from build123d import *

# Parameters (mm, degrees)
CROQUIS3_R              = 0.5
CORTAR_EXTRUIR1_DEPTH   = 1
SALIENTE_EXTRUIR3_START = 5
SALIENTE_EXTRUIR3_DEPTH = 5


with BuildPart() as part:
    # Croquis2 → Revolución1 (revolve)
    with BuildSketch(Plane(origin=(0, 0, 0), x_dir=(0, 0, -1), z_dir=(1, 0, 0)), mode=Mode.PRIVATE) as revoluci_n1_sk:
        Polygon((0, 0), (0, 6.5), (-0.95, 6.5), (-0.95, 6.4), (-1.05, 6.4), (-1.05, 6.5), (-4, 6.5), (-4, 3.5), (-5, 3.5), (-5, 2), (-8, 2), (-8, 1.75), (-4, 1.75), (-4, 0), align=None)
    revolve(revoluci_n1_sk.sketch.rotate(Axis((0, 0, 4), (0, 0, -1)), 90), axis=Axis((0, 0, 4), (0, 0, -1)))

    # Croquis3 → Cortar-Extruir1 (cut)
    with BuildSketch(Plane(origin=(0, 0, 0), x_dir=(-1, 0, 0), z_dir=(0, 0, -1))):
        with Locations((-2, -3)):
            Circle(CROQUIS3_R)
        with Locations((2, -3)):
            Circle(CROQUIS3_R)
        with Locations((0, -2)):
            Circle(CROQUIS3_R)
    extrude(amount=-CORTAR_EXTRUIR1_DEPTH, mode=Mode.SUBTRACT)

    # Croquis5 → Saliente-Extruir3 (add)
    with BuildSketch(Plane(origin=(0, 0, 1), x_dir=(-1, 0, 0), z_dir=(0, 0, -1)).offset(SALIENTE_EXTRUIR3_START)):
        with BuildLine():
            Line((-0.489897949, -1.9), (0.489897949, -1.9))
            ThreePointArc((0.489897949, -1.9), (0.5, -2), (0.489897949, -2.1))
            Line((0.489897949, -2.1), (-0.489897949, -2.1))
            ThreePointArc((-0.489897949, -2.1), (-0.5, -2), (-0.489897949, -1.9))
        make_face()
        with BuildLine():
            Line((1.510102051, -2.9), (2.489897949, -2.9))
            ThreePointArc((2.489897949, -2.9), (2.5, -3), (2.489897949, -3.1))
            Line((2.489897949, -3.1), (1.510102051, -3.1))
            ThreePointArc((1.510102051, -3.1), (1.5, -3), (1.510102051, -2.9))
        make_face()
        with BuildLine():
            Line((-2.489897949, -2.9), (-1.510102051, -2.9))
            ThreePointArc((-1.510102051, -2.9), (-1.5, -3), (-1.510102051, -3.1))
            Line((-1.510102051, -3.1), (-2.489897949, -3.1))
            ThreePointArc((-2.489897949, -3.1), (-2.5, -3), (-2.489897949, -2.9))
        make_face()
    extrude(amount=-SALIENTE_EXTRUIR3_DEPTH)


solid = part.part
For this review, take the finished solid that the model builds, in its own axes (mm). A direction names the side the tool comes from. Round coordinates to 2 decimals unless told otherwise and drop trailing zeros. Loops run counter-clockwise (first coordinate to the right, second up) from the corner with the lowest first, then second, coordinate; pieces in that order, holes last. Notation, with made-up numbers: (64.5, -28.75) - (74.5, -28.75) arc R17 ccw to (74.5, -20.75) - close; hole circle Ø6 at (37.5, 32). An arc over 180 degrees is marked (long way). One line per item, written item: value. Start each with the question number.
Item 1: For faces 1 (the flat face through (2, -2.9, -2)), 2 (the flat face through (0, 0, 4)), list the 3-axis set-ups (+Z, -Z, +X, -X, +Y, -Y) from which the entire face can be reached by the end or side of a thin tool; tool diameter is ignored.
Item 2: Take a section at A-A (z = 0.25). Give the boundary of the cut face in (x, y).
Item 3: The part is to be moulded in two halves that separate along Y. For faces 3 (the flat face through (0, 0, 0)), 4 (the flat face through (0, -2.1, -2)), 5 (the cylindrical face through (-2, -2.5, 0.5)), 6 (the cylindrical face through (-5.158, 3.955, 0.482)), say which applies: +Y half, -Y half, draft (parallel to the pull), parting line (faces both ways), or undercut.
Item 4: Take a section at B-B (y = 0). Give the boundary of the cut face in (x, z), plus the area to 3 significant figures.
Item 5: Clearance check with flat-ended pins moving along their axes: pin 1 Ø5 at (x, z) = (5, 1) entering from +Y; pin 2 Ø1.5 at (x, z) = (-3, -1.5) entering from +Y; pin 3 Ø1.1 at (x, z) = (0, -2) entering from +Y. State where each tip first meets the part, or that it passes through.
Item 6: For L1, parallel to Y at x = 0, z = 6.2; L2, parallel to Y at x = 0, z = 4.9; L3, parallel to Z at x = -3.5, y = 5.25, list the stretches that pass through material, from the lowest coordinate up.
Item 7: Take a section at C-C (x = 0.75). Give the boundary of the cut face in (y, z).
Item 8: Take a section at D-D (z = 5.5). Give the boundary of the cut face in (x, y).
Answer below:
1. face 1: -Z
1. face 2: +Z
2. outline: circle Ø13 at (0, 0); hole (-2.49, -3.1) arc R0.5 ccw to (-1.51, -3.1) - close; hole (-2.49, -2.9) - (-1.51, -2.9) arc R0.5 ccw to start; hole (-0.49, -2.1) arc R0.5 ccw to (0.49, -2.1) - close; hole (-0.49, -1.9) - (0.49, -1.9) arc R0.5 ccw to start; hole (1.51, -3.1) arc R0.5 ccw to (2.49, -3.1) - close; hole (1.51, -2.9) - (2.49, -2.9) arc R0.5 ccw to start
3. face 3: draft
3. face 4: undercut
3. face 5: undercut
3. face 6: parting line
4. outline: (-6.5, 0) - (6.5, 0) - (6.5, 0.95) - (6.4, 0.95) - (6.4, 1.05) - (6.5, 1.05) - (6.5, 4) - (3.5, 4) - (3.5, 5) - (2, 5) - (2, 8) - (1.75, 8) - (1.75, 4) - (-1.75, 4) - (-1.75, 8) - (-2, 8) - (-2, 5) - (-3.5, 5) - (-3.5, 4) - (-6.5, 4) - (-6.5, 1.05) - (-6.4, 1.05) - (-6.4, 0.95) - (-6.5, 0.95) - close
4. area: 57.0 mm2
5. pin 1: stops at y = 6
5. pin 2: stops at y = -2.9
5. pin 3: stops at y = -1.9
6. L1: y = -2 to -1.75, 1.75 to 2
6. L2: y = -3.5 to -1.75, 1.75 to 3.5
6. L3: z = 0 to 4
7. outline: (-6.46, 0) - (6.46, 0) - (6.46, 0.95) - (6.36, 0.95) - (6.36, 1.05) - (6.46, 1.05) - (6.46, 4) - (3.42, 4) - (3.42, 5) - (1.85, 5) - (1.85, 8) - (1.58, 8) - (1.58, 4) - (-1.58, 4) - (-1.58, 8) - (-1.85, 8) - (-1.85, 5) - (-3.42, 5) - (-3.42, 4) - (-6.46, 4) - (-6.46, 1.05) - (-6.36, 1.05) - (-6.36, 0.95) - (-6.46, 0.95) - close
8. outline: circle Ø4 at (0, 0); hole circle Ø3.5 at (0, 0)
